Verification items for this drawing (mm, ordinates from the low corner). A direction names the side the tool comes from. Round coordinates to 2 decimals unless told otherwise and drop trailing zeros. Write each loop counter-clockwise with the first axis right and the second up, starting at its lowest first coordinate (ties: lowest second). Pieces come first, ordered by that corner, then holes.
Item 1: Cross-section at D-D (z = 4). Enter the section's corners in (x, y).
Item 2: Cross-section at B-B (z = 26). Enter the section's corners in (x, y) (3 decimals).
Item 3: Cross-section at C-C (y = 76). Enter the section's corners in (x, z), then the cut area to 3 significant figures.
Item 4: Depth check by flat-ended pin: P1, Ø6, axis at x = 11.5, y = 84, coming from the -Z side; P2, Ø9.5, axis at x = 8.5, y = 81, coming from the +Z side; P3, Ø5, axis at x = 14, y = 97, coming from the +Z side; P4, Ø5, axis at x = 17, y = 102.5, coming from the -Z side. Enter the tip coordinate at first touch or a pass-through.
Item 5: Cross-section at A-A (x = 10). Enter the section's corners in (y, z) (3 decimals), then the cut area to 3 significant figures.
Item 6: Access from +Z, -Z, +X, -X, +Y, -Y to the whole of each face (thin tool, end or side, straight path). Record for the marked faces 1, 2, 3 and 4.
Item 7: Scan lines: probe 1 along Y at (x, z) = (7.5, 2.5); probe 2 along Y at (x, z) = (15, 25); probe 3 along Z at (x, y) = (11, 80.5). Record each from-to range of solid material in increasing order.
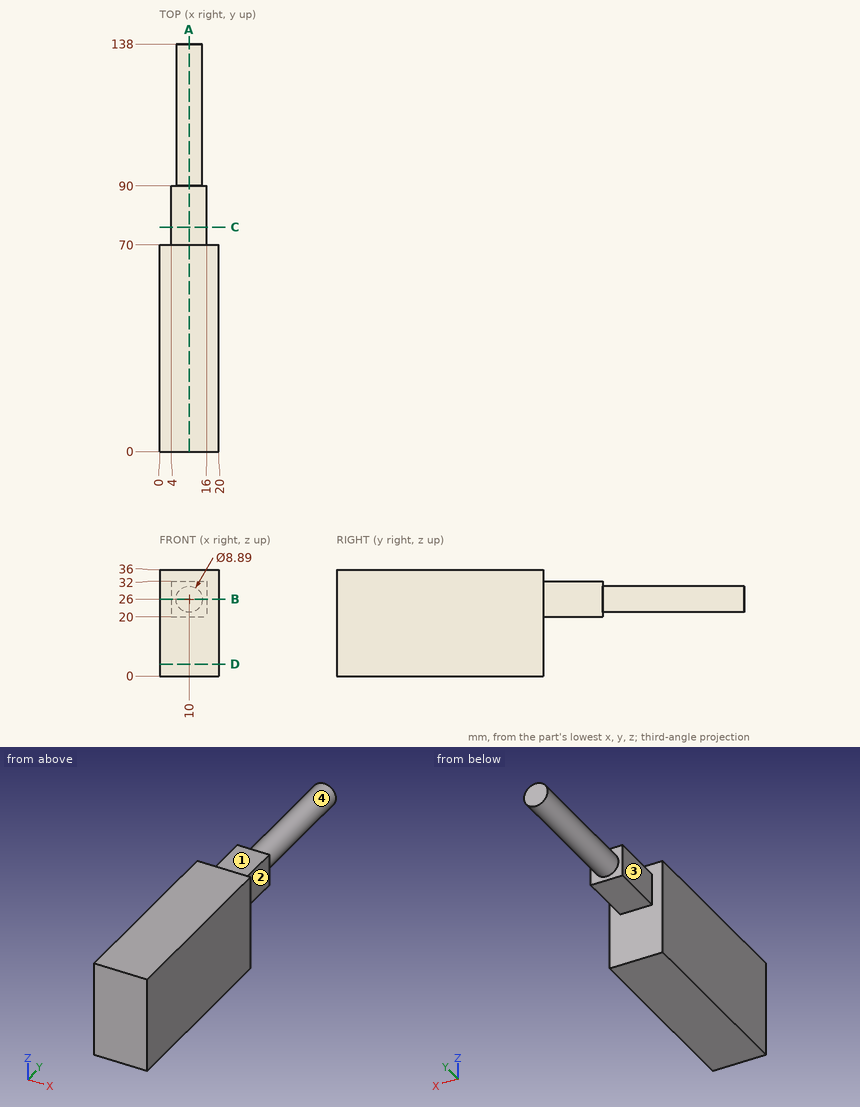
Resolved:
1. outline: (0, 0) - (20, 0) - (20, 70) - (0, 70) - close
2. outline: (0, 0) - (20, 0) - (20, 70) - (16, 70) - (16, 90) - (14.445, 90) - (14.445, 138) - (5.555, 138) - (5.555, 90) - (4, 90) - (4, 70) - (0, 70) - close
3. outline: (4, 20) - (16, 20) - (16, 32) - (4, 32) - close
3. area: 144 mm2
4. P1: stops at z = 20
4. P2: stops at z = 32
4. P3: stops at z = 30.18
4. P4: passes through
5. outline: (0, 0) - (70, 0) - (70, 20) - (90, 20) - (90, 21.555) - (138, 21.555) - (138, 30.445) - (90, 30.445) - (90, 32) - (70, 32) - (70, 36) - (0, 36) - close
5. area: 3,190 mm2
6. face 1: +Z, +X, -X, +Y
6. face 2: +Z, -Z, +X, +Y
6. face 3: +Z, -Z, -X, +Y
6. face 4: +Y
7. probe 1: y = 0 to 70
7. probe 2: y = 0 to 90
7. probe 3: z = 20 to 32
